Part print with two shaded views. Sizes in mm from the minimum x, y, z corner. Round coordinates to 2 decimals unless told otherwise and drop trailing zeros. Write each loop counter-clockwise with the first axis right and the second up, starting at its lowest first coordinate (ties: lowest second). Pieces come first, ordered by that corner, then holes. Notation, with made-up numbers: M 88,-2.5 L 131,-2.5 A34 ccw 131,27.5 Z; hole C 43.25,10 d3. An arc over 180 degrees is marked long. One line per question, with ' | ' between items. Start each with the question number.
1) Saw through at D-D (y = 468.5). List the corners of the cut face in (x, z), plus the area to 3 significant figures.
2) Mould opens along Y. For the marked faces 1, 2 and 3 say: pulls with the +Y half, pulls with the -Y half, needs draft (parallel to the pull), parting line crosses it, or undercut.
3) Saw through at A-A (z = 124.5). List the corners of the cut face in (x, y).
4) Saw through at C-C (x = 467.5). List the corners of the cut face in (y, z), plus the area to 3 significant figures.
5) Drop flat-ended pins along their axis: pin 1 Ø1.5 at (x, y) = (365.5, 328) entering from -Z; pin 2 Ø7.5 at (x, z) = (156.5, 170) entering from -Y. Give the stop position or say it passes through.
6) Saw through at B-B (y = 40.5). List the corners of the cut face in (x, z).
7) Wall check: probe 1 along X at (y, z) = (54, 86); probe 2 along Z at (x, y) = (88, 442.5); probe 3 along Y at (x, z) = (52, 57). Give the ranges that are in metal, low to high. Write a range as [from, to].
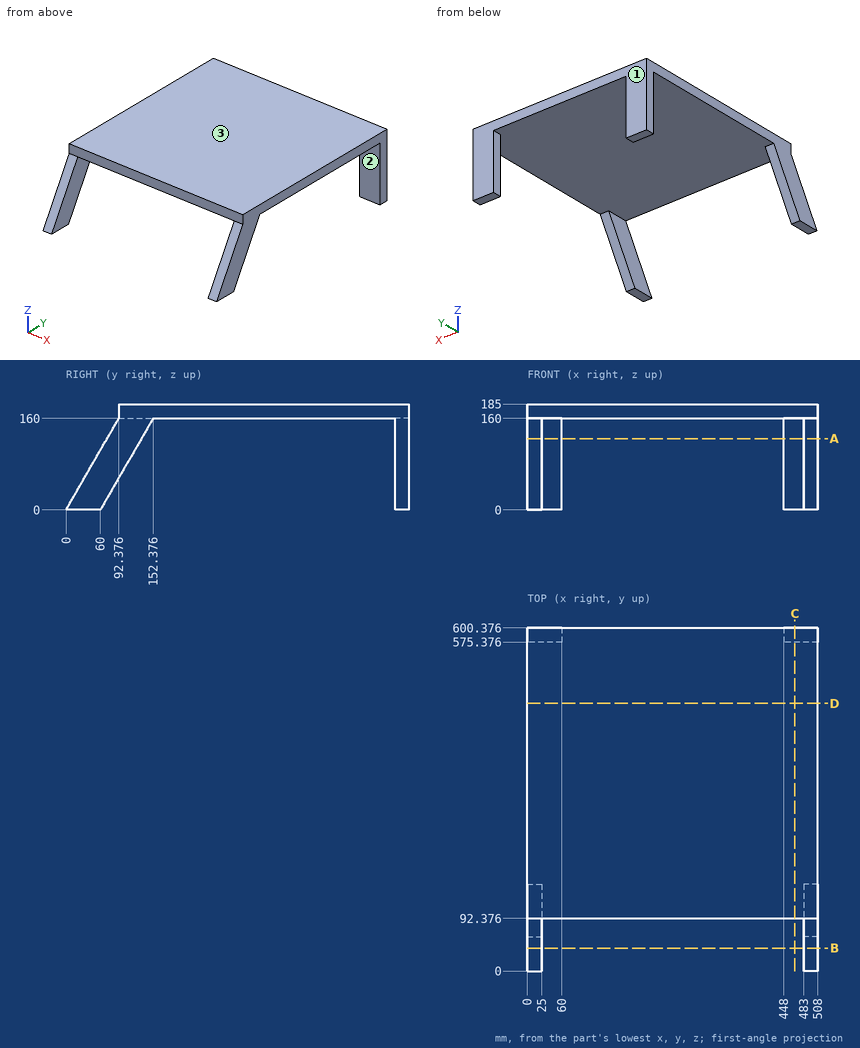
Answer key:
1) outline: M 0,160 L 508,160 L 508,185 L 0,185 Z | area: 12,700 mm2
2) face 1: pulls with the +Y half | face 2: undercut | face 3: needs draft
3) outline: M 0,71.88 L 25,71.88 L 25,131.88 L 0,131.88 Z; M 0,575.38 L 60,575.38 L 60,600.38 L 0,600.38 Z; M 448,575.38 L 508,575.38 L 508,600.38 L 448,600.38 Z; M 483,71.88 L 508,71.88 L 508,131.88 L 483,131.88 Z
4) outline: M 92.38,160 L 575.38,160 L 575.38,0 L 600.38,0 L 600.38,185 L 92.38,185 Z | area: 16,700 mm2
5) pin 1: stops at z = 160 | pin 2: stops at y = 92.38
6) outline: M 0,0 L 25,0 L 25,70.15 L 0,70.15 Z; M 483,0 L 508,0 L 508,70.15 L 483,70.15 Z
7) probe 1: x = [0, 25], [483, 508] | probe 2: z = [160, 185] | probe 3: y = [575.38, 600.38]
